Source: three-view drawing plus pictorial views. Frame: mm from the lowest corner of the part. Round coordinates to 2 decimals unless told otherwise and drop trailing zeros. Loops run counter-clockwise (first coordinate to the right, second up) from the corner with the lowest first, then second, coordinate; pieces in that order, holes last. Notation, with made-up numbers: (52, 18.25) -> (66, 18.25) arc R9 cw to (66, 31.25) -> close; hole circle Ø9 at (-27.5, -26). An arc over 180 degrees is marked (long way). Answer in a Markdown table with one row per item. Add a question column.
Q1. Section B-B, the plane x = 42. Output: boundary loops of the cut face in (y, z), and give its area (3 significant figures).
Q2. Section C-C, the plane x = 7.5. Output: boundary loops of the cut face in (y, z), and give its area (3 significant figures).
Q3. Section A-A, the plane y = 95. Output: boundary loops of the cut face in (x, z), and give its area (3 significant figures).
Q4. Pin query (flat end, axial travel): pin 1 (4 mm diameter, centred on x = 152.5, y = 95, fed in from +Z). Return the tip coordinate at first contact, or that it passes through.
Q5. Section D-D, the plane z = 1.05. Give the number of separate pieces and of enclosed holes in the cut face, and give its area (3 significant figures).
Q6. Ray query, L1, parallel to Y at x = 152.5, z = 1.15; L2, parallel to X at y = 95, z = 1.45; L3, parallel to Y at x = 80, z = 1.45. Return the intervals inside material, ascending. Write a range as from..to.
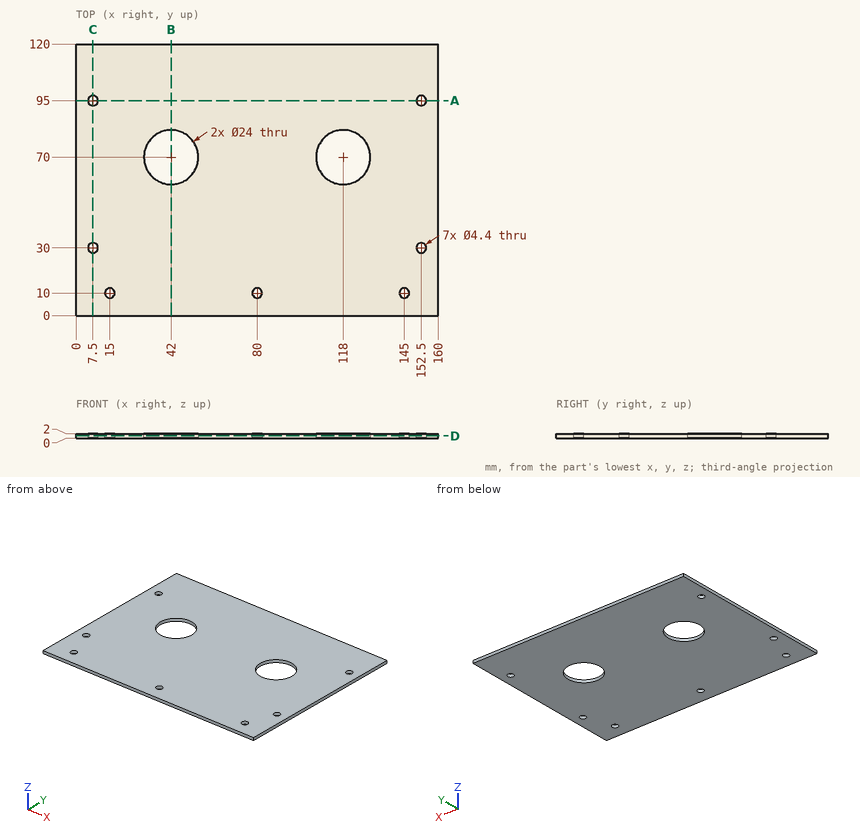
Answer block:
| question | item | result |
|---|---|---|
| 1 | outline | (0, 0) -> (58, 0) -> (58, 2) -> (0, 2) -> close; (82, 0) -> (120, 0) -> (120, 2) -> (82, 2) -> close |
| 1 | area | 192 mm^2 |
| 2 | outline | (0, 0) -> (27.8, 0) -> (27.8, 2) -> (0, 2) -> close; (32.2, 0) -> (92.8, 0) -> (92.8, 2) -> (32.2, 2) -> close; (97.2, 0) -> (120, 0) -> (120, 2) -> (97.2, 2) -> close |
| 2 | area | 222 mm^2 |
| 3 | outline | (0, 0) -> (5.3, 0) -> (5.3, 2) -> (0, 2) -> close; (9.7, 0) -> (150.3, 0) -> (150.3, 2) -> (9.7, 2) -> close; (154.7, 0) -> (160, 0) -> (160, 2) -> (154.7, 2) -> close |
| 3 | area | 302 mm^2 |
| 4 | pin 1 | through |
| 5 | separate pieces | 1 |
| 5 | enclosed holes | 9 |
| 5 | area | 18,200 mm^2 |
| 6 | L1 | 0..27.8, 32.2..92.8, 97.2..120 |
| 6 | L2 | 0..5.3, 9.7..150.3, 154.7..160 |
| 6 | L3 | 0..7.8, 12.2..120 |
